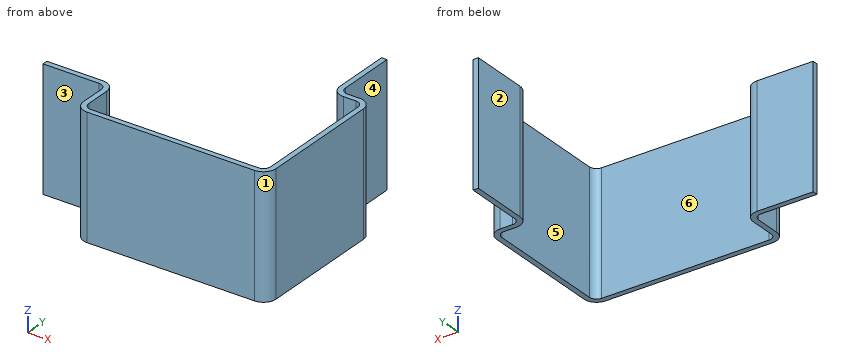
from build123d import *

# Parameters (mm, degrees)
BRIDA_BASE1_DEPTH = 144.15


# Sheet-metal steps are written as plain solids
with BuildPart() as part:
    # Croquis1 → Brida base1 (new body)
    with BuildSketch(Plane.XY):
        with BuildLine():
            Line((258.7, 246.05), (258.7, 176.93))
            ThreePointArc((258.7, 176.93), (263.058251096, 166.408251096), (273.58, 162.05))
            Line((273.58, 162.05), (288.17, 162.05))
            ThreePointArc((288.17, 162.05), (294.201620844, 159.551620844), (296.7, 153.52))
            Line((296.7, 153.52), (296.7, 8.53))
            ThreePointArc((296.7, 8.53), (294.201620844, 2.498379156), (288.17, 0))
            Line((288.17, 0), (89.93, 0))
            ThreePointArc((89.93, 0), (83.898379156, 2.498379156), (81.4, 8.53))
            Line((81.4, 8.53), (81.4, 38.12))
            ThreePointArc((81.4, 38.12), (77.041748904, 48.641748904), (66.52, 53))
            Line((66.52, 53), (0, 53))
            Line((0, 53), (0, 46.65))
            Line((0, 46.65), (66.52, 46.65))
            ThreePointArc((66.52, 46.65), (72.551620844, 44.151620844), (75.05, 38.12))
            Line((75.05, 38.12), (75.05, 8.53))
            ThreePointArc((75.05, 8.53), (79.408251096, -1.991748904), (89.93, -6.35))
            Line((89.93, -6.35), (288.17, -6.35))
            ThreePointArc((288.17, -6.35), (298.691748904, -1.991748904), (303.05, 8.53))
            Line((303.05, 8.53), (303.05, 153.52))
            ThreePointArc((303.05, 153.52), (298.691748904, 164.041748904), (288.17, 168.4))
            Line((288.17, 168.4), (273.58, 168.4))
            ThreePointArc((273.58, 168.4), (267.548379156, 170.898379156), (265.05, 176.93))
            Line((265.05, 176.93), (265.05, 246.05))
            Line((265.05, 246.05), (258.7, 246.05))
        make_face()
    extrude(amount=BRIDA_BASE1_DEPTH)


solid = part.part
Model file for the job. Use its own axes, mm. Face numbers are marked on the shaded views. A direction names the side the tool comes from. Give positions to 0.01 mm unless a question says otherwise; leave off trailing zeros. Loops run counter-clockwise (first coordinate to the right, second up) from the corner with the lowest first, then second, coordinate; pieces in that order, holes last.
1) Saw through at B-B (x = 269.5). Write the cut outline in (y, z), plus the area to 3 significant figures.
2) Pull direction X, two halves, no side cores. Call the marked faces 3, 4, 5 and 6: +X half, -X half, draft (parallel to the pull), parting line (faces both ways), or undercut.
3) Saw through at A-A (y = 18). Write the cut outline in (x, z).
4) Wall check: line 1 (X direction, y = 18, z = 107); line 2 (Y direction, x = 189, z = 112); line 3 (X direction, y = 183, z = 111.5). Give the ranges that are in metal, low to high.
5) Saw through at C-C (z = 33.5). Write the cut outline in (x, y), plus the area to 3 significant figures.
6) Tool access for the marked faces 1 and 2: list every direction of +Z, -Z, +X, -X, +Y, -Y with a clear straight run to the whole face (end or side of a thin tool).
7) Saw through at D-D (y = 104). Write the cut outline in (x, z).
8) Flat gauge pins, fed straight in: pin 1 Ø1 at (x, z) = (196, 95.5) entering from +Y; pin 2 Ø6 at (y, z) = (174.5, 71.5) entering from +X; pin 3 Ø7.5 at (x, z) = (280, 98) entering from +Y; pin 4 Ø12 at (y, z) = (56.5, 91) entering from -X. Where does each tip first touch, or does it go through?
Answer block:
1. outline: (-6.35, 0) - (0, 0) - (0, 144.15) - (-6.35, 144.15) - close; (162.62, 0) - (169.44, 0) - (169.44, 144.15) - (162.62, 144.15) - close
1. area: 1,900 mm2
2. face 3: draft
2. face 4: +X half
2. face 5: undercut
2. face 6: undercut
3. outline: (75.05, 0) - (81.4, 0) - (81.4, 144.15) - (75.05, 144.15) - close; (296.7, 0) - (303.05, 0) - (303.05, 144.15) - (296.7, 144.15) - close
4. line 1: x = 75.05 to 81.4, 296.7 to 303.05
4. line 2: y = -6.35 to 0
4. line 3: x = 258.7 to 265.05
5. outline: (0, 46.65) - (66.52, 46.65) arc R8.53 cw to (75.05, 38.12) - (75.05, 8.53) arc R14.88 ccw to (89.93, -6.35) - (288.17, -6.35) arc R14.88 ccw to (303.05, 8.53) - (303.05, 153.52) arc R14.88 ccw to (288.17, 168.4) - (273.58, 168.4) arc R8.53 cw to (265.05, 176.93) - (265.05, 246.05) - (258.7, 246.05) - (258.7, 176.93) arc R14.88 ccw to (273.58, 162.05) - (288.17, 162.05) arc R8.53 cw to (296.7, 153.52) - (296.7, 8.53) arc R8.53 cw to (288.17, 0) - (89.93, 0) arc R8.53 cw to (81.4, 8.53) - (81.4, 38.12) arc R14.88 ccw to (66.52, 53) - (0, 53) - close
5. area: 3,910 mm2
6. face 1: +Z, -Z, +X, -Y
6. face 2: +Z, -Z, -X, +Y
7. outline: (296.7, 0) - (303.05, 0) - (303.05, 144.15) - (296.7, 144.15) - close
8. pin 1: stops at y = 0
8. pin 2: stops at x = 267
8. pin 3: stops at y = 168.4
8. pin 4: stops at x = 0
